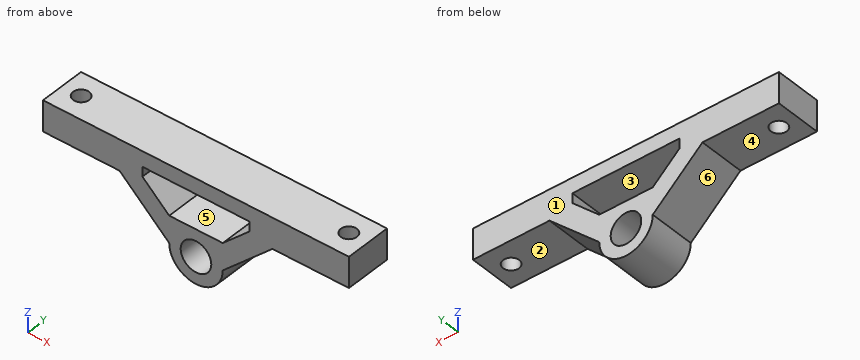
from build123d import *

# Parameters (mm, degrees)
SKETCH_1_R            = 4
EXTRUDE_1_DEPTH       = 12
HOLE_WIZARD_M41_D     = 4.2
HOLE_WIZARD_M41_DEPTH = 8
HOLE_WIZARD_M41_TIP   = 1.2618073


with BuildPart() as part:
    # Эскиз1 → Бобышка-Вытянуть1 (new body)
    with BuildSketch(Plane(origin=(0, 0, 0), x_dir=(1, 0, 0), z_dir=(0, 1, 0))):
        with BuildLine():
            Line((-40, -20), (40, -20))
            Line((40, -20), (40, -12))
            Line((40, -12), (20, -12))
            Line((20, -12), (7, 0))
            ThreePointArc((7, 0), (0, 7), (-7, 0))
            Line((-7, 0), (-20, -12))
            Line((-20, -12), (-40, -12))
            Line((-40, -12), (-40, -20))
        make_face()
        Circle(SKETCH_1_R, mode=Mode.SUBTRACT)
        Polygon((-14, -16), (14, -16), (14, -13.461538462), (7, -7), (-7, -7), (-14, -13.461538462), align=None, mode=Mode.SUBTRACT)
    extrude(amount=EXTRUDE_1_DEPTH)

    # Сверло под метчик  спиральное M41
    with Locations(Plane.XY.offset(20)):
        with Locations((-35, 6), (35, 6)):
            Hole(HOLE_WIZARD_M41_D / 2, depth=HOLE_WIZARD_M41_DEPTH)
            with Locations((0, 0, -(HOLE_WIZARD_M41_DEPTH + HOLE_WIZARD_M41_TIP / 2))):  # 118° drill point
                Cone(0, HOLE_WIZARD_M41_D / 2, HOLE_WIZARD_M41_TIP, mode=Mode.SUBTRACT)


solid = part.part
Here's how the part is built. I have some questions about the finished solid (model axes, mm). Face numbers are marked on the shaded views. A direction names the side the tool comes from. Coordinates: 2 decimals unless noted, no trailing zeros. Order: outer loops, then holes, each group sorted by start corner. A loop starts at its lowest first (then second) coordinate and runs counter-clockwise, first axis right, second up. Notation, with made-up numbers: (-11, 36.5) -> (2, 36.5) arc R16 ccw to (2, 61.5) -> close; hole circle Ø7 at (7, 40.5). An arc over 180 degrees is marked (long way). Answer in a Markdown table with one row per item.
(1) I want a section at B-B on x = 0. List the corners of the cut face in (y, z) for me, then the cut area to 3 significant figures.
Answer key:
| item | result |
|---|---|
| outline | (0, -7) -> (12, -7) -> (12, -4) -> (0, -4) -> close; (0, 4) -> (12, 4) -> (12, 7) -> (0, 7) -> close; (0, 16) -> (12, 16) -> (12, 20) -> (0, 20) -> close |
| area | 120 mm^2 |
(2) Please list where these lines run through material, in increasing order: probe 1 along Z at (x, y) = (0, 5); probe 2 along Y at (x, z) = (35, 16.75); probe 3 along Z at (x, y) = (33, 1).
Answer key:
| item | result |
|---|---|
| probe 1 | -7 to -4, 4 to 7, 16 to 20 |
| probe 2 | 0 to 3.9, 8.1 to 12 |
| probe 3 | 12 to 20 |
(3) I want a section at A-A on z = 14.5. List the corners of the cut face in (x, y) for me.
Answer key:
| item | result |
|---|---|
| outline | (-40, 0) -> (-14, 0) -> (-14, 12) -> (-40, 12) -> close; (14, 0) -> (40, 0) -> (40, 12) -> (14, 12) -> close; hole circle Ø4.2 at (-35, 6); hole circle Ø4.2 at (35, 6) |
(4) Thinking about a two-plate mould opening in X: for the marked faces 4, 5 and 6, which applies, +X half, -X half, draft (parallel to the pull), parting line (faces both ways), or undercut?
Answer key:
| item | result |
|---|---|
| face 4 | draft |
| face 5 | undercut |
| face 6 | -X half |
(5) On a 3-axis mill with a long thin cutter (end or side, diameter ignored), from which of +Z, -Z, +X, -X, +Y, -Y can I reach the whole of each face in a straight line? I mean the marked faces 1, 2 and 3. Say none if no direction works.
Answer key:
| item | result |
|---|---|
| face 1 | +Z, -Z, +X, -X, +Y |
| face 2 | -Z, +X, +Y, -Y |
| face 3 | +Y, -Y |
(6) I want a section at D-D on y = 1. List the corners of the cut face in (x, z) for me, then the cut area to 3 significant figures.
Answer key:
| item | result |
|---|---|
| outline | (-40, 12) -> (-20, 12) -> (-7, 0) arc R7 ccw to (7, 0) -> (20, 12) -> (40, 12) -> (40, 20) -> (-40, 20) -> close; hole (-14, 13.46) -> (-7, 7) -> (7, 7) -> (14, 13.46) -> (14, 16) -> (-14, 16) -> close; hole circle Ø8 at (0, 0) |
| area | 784 mm^2 |
(7) I want a section at C-C on x = 35. List the corners of the cut face in (y, z) for me, then the cut area to 3 significant figures.
Answer key:
| item | result |
|---|---|
| outline | (0, 12) -> (3.9, 12) -> (3.9, 20) -> (0, 20) -> close; (8.1, 12) -> (12, 12) -> (12, 20) -> (8.1, 20) -> close |
| area | 62.4 mm^2 |
(8) Will these pins go through, and if not, where does the flat tip stop? pin 1 Ø5 at (x, y) = (-4, 1.5) entering from -Z; pin 2 Ø3.5 at (x, y) = (-32.5, 6.5) entering from -Z; pin 3 Ø5 at (y, z) = (4, 4) entering from -X.
Answer key:
| item | result |
|---|---|
| pin 1 | z = -6.84 |
| pin 2 | z = 12 |
| pin 3 | x = -14.04 |
